Verification items for the finished model (mm, model axes). A direction names the side the tool comes from. Coordinates: 2 decimals unless noted, no trailing zeros. Write each loop counter-clockwise with the first axis right and the second up, starting at its lowest first coordinate (ties: lowest second). Pieces come first, ordered by that corner, then holes. Notation, with made-up numbers: M 15,2 L 50,2 A26 ccw 50,19 Z; hole C -20.5,-25.75 d8. An arc over 180 degrees is marked long. One line per item, written item: value.
```python
from build123d import *

# Parameters (mm, degrees)
CUT_EXTRUDE1_DEPTH = 2.9765625
CHAMFER1_SIZE      = 0.396875
CHAMFER2_SIZE      = 0.1984375


with BuildPart() as part:
    # Sketch2 → Revolve1 (revolve)
    with BuildSketch(Plane(origin=(0, 0, 0), x_dir=(0, 0, -1), z_dir=(1, 0, 0)), mode=Mode.PRIVATE) as revolve1_sk:
        Polygon((11.938, 1.8176875), (11.3426875, 2.413), (-7.112, 2.413), (-7.112, 3.96875), (-11.938, 3.96875), (-11.938, 0), (11.938, 0), align=None)
    revolve(revolve1_sk.sketch.rotate(Axis((0, 0, -11.938), (0, 0, 1)), 90), axis=Axis((0, 0, -11.938), (0, 0, 1)))

    # Sketch4 → Cut-Extrude1 (cut)
    with BuildSketch(Plane.XY.offset(11.938)):
        Polygon((0, 2.291358881), (-1.984375, 1.14567944), (-1.984375, -1.14567944), (0, -2.291358881), (1.984375, -1.14567944), (1.984375, 1.14567944), align=None)
    extrude(amount=-CUT_EXTRUDE1_DEPTH, mode=Mode.SUBTRACT)

    # Cut-Extrude2 cone 1 section (on through the dimple's axis) → Cut-Extrude2 (revolve, cut)
    with BuildSketch(Plane(origin=(0, 0, 11.938), x_dir=(0, -1, 0), z_dir=(1, 0, 0))):
        Polygon((0, 0), (2.291358881, 0), (0, 1.322916667), align=None)
    revolve(axis=Axis((0, 0, 11.938), (0, 0, -1)), mode=Mode.SUBTRACT)

    # Chamfer1
    chamfer1_edges = [part.edges().sort_by_distance(p)[0] for p in [
        (3.96875, 0, 11.938),
    ]]
    chamfer(chamfer1_edges, length=CHAMFER1_SIZE)

    # Chamfer2
    chamfer2_edges = [part.edges().sort_by_distance(p)[0] for p in [
        (3.96875, 0, 7.112),
    ]]
    chamfer(chamfer2_edges, length=CHAMFER2_SIZE)


solid = part.part
```
Item 1: Scan lines: line 1 (Z direction, x = 0.25, y = -2.5); line 2 (Y direction, x = -0.75, z = 2.75); line 3 (Z direction, x = -1, y = 0.75). Record each from-to range of solid material in increasing order.
The answers:
line 1: z = 7.11 to 11.94
line 2: y = -2.29 to 2.29
line 3: z = -11.94 to 8.96
Item 2: Go/stop test with flat-tipped pins: P1, Ø3, axis at x = -2, y = 2, coming from the -Z side; P2, Ø3, axis at y = 2.5, z = 7.5, coming from the -X side; P3, Ø1, axis at x = 1, z = -8.5, coming from the -Y side. Record where each tip stops, or that it passes through.
The answers:
P1: stops at z = -11.94
P2: stops at x = -3.84
P3: stops at y = -2.36
Item 3: Cross-section at A-A, the plane z = 10.5. Enter the section's corners in (x, y).
The answers:
outline: C 0,0 d7.94; hole M -1.98,-1.15 L 0,-2.29 L 1.98,-1.15 L 1.98,1.15 L 0,2.29 L -1.98,1.15 Z
Item 4: Access from +Z, -Z, +X, -X, +Y, -Y to the whole of each face (thin tool, end or side, straight path). Record for faces 1 (the face through (-1.081, 1.842, 11.848)), 2 (the face through (-0.74, 2.33, 11.938)), 3 (the face through (2.5, 0.8, 7.112)).
The answers:
face 1: +Z
face 2: +Z, +X, -X, +Y, -Y
face 3: -Z
Item 5: Draft check along X on faces 4 (the face through (-1.01, -1.71, 10.47)), 5 (the face through (0, 0, -11.938)), 6 (the face through (1.915, 1.468, -1.986)). Enter one of: released by +X, released by -X, zero draft, split by the parting line, or undercut.
The answers:
face 4: undercut
face 5: zero draft
face 6: split by the parting line
Item 6: Cross-section at B-B, the plane y = 0. Enter the section's corners in (x, z).
The answers:
outline: M -3.97,7.31 L -3.77,7.11 L -2.41,7.11 L -2.41,-11.34 L -1.82,-11.94 L 1.82,-11.94 L 2.41,-11.34 L 2.41,7.11 L 3.77,7.11 L 3.97,7.31 L 3.97,11.54 L 3.57,11.94 L 2.29,11.94 L 1.98,11.76 L 1.98,8.96 L -1.98,8.96 L -1.98,11.76 L -2.29,11.94 L -3.57,11.94 L -3.97,11.54 Z
Item 7: Cross-section at C-C, the plane z = -3.75. Enter the section's corners in (x, y).
The answers:
outline: C 0,0 d4.83
